Model file for the job. Use its own axes, mm. A direction names the side the tool comes from. Round coordinates to 2 decimals unless told otherwise and drop trailing zeros. Write each loop counter-clockwise with the first axis right and the second up, starting at its lowest first coordinate (ties: lowest second). Pieces come first, ordered by that corner, then holes.
Autodesk Inventor part; units mm, degrees
ref_plane "YZ Plane" through (0, 0, 0) normal (1, 0, 0) x (0, 1, 0)
ref_plane "XZ Plane" through (0, 0, 0) normal (0, 1, 0) x (-1, 0, 0)
ref_plane "XY Plane" through (0, 0, 0) normal (0, 0, 1) x (1, 0, 0)
sketch "Sketch1" plane through (0, 0, 0) normal (0, 0, 1) x (1, 0, 0)
  line L0 (0, 0) -> (50, 0)
  line L1 (50, 0) -> (50, 50)
  line L2 (50, 50) -> (0, 50)
  line L3 (0, 13.5853) -> (5.2, 11.6926)
  line L4 (5.2, 11.6926) -> (5.2, 22.0926)
  line L5 (5.2, 22.0926) -> (0, 20.2)
  line L6 (0, 50) -> (0, 20.2)
  line L7 (0, 13.5853) -> (0, 0)
  line L8 (0, 40.2) -> (5.2, 42.0926)
  line L9 (5.2, 42.0926) -> (5.2, 31.6926)
  line L10 (5.2, 31.6926) -> (0, 33.5853)
  dimension "d0" = 50
  dimension "d1" = 50
  dimension "d2" = 50
  dimension "d8" = 10.4
  dimension "d9" = 70
  dimension "d10" = 70
  dimension "d11" = 20.2
  dimension "d12" = 5.2
  dimension "d13" = 5.2
  dimension "d14" = 10.4
  dimension "d15" = 40.2
  dimension "d16" = 70
  dimension "d17" = 70
  dimension "d18" = 6.6147
  dimension "d19" = 6.6147
  dimension "d26" = 13.5853
extrude "Extrusion1" add sketch "Sketch1" along normal blind 10 contours L7 L3 L4 L5 L6 L10 L9 L8 L2 L1 L0
sketch "Sketch2" plane through (0, 0, 10) normal (0, 0, 1) x (1, 0, 0)
  line L0 (0, 13.5853) -> (0, 0)
  line L1 (0, 0) -> (50, 0)
  line L2 (50, 0) -> (50, 6.2593)
  line L3 (50, 0) -> (50, 50)
  line L4 (0, 0) -> (0, 6.2593)
  line L5 (0, 0) -> (50, 0)
  line L6 (0, 6.2593) -> (50, 6.2593)
  circle A0 centre (25, 25) radius 2.8
  dimension "d23" = 5.6
extrude "Extrusion2" add sketch "Sketch2" along normal blind 45
sketch "Sketch3" plane through (0, 0, 0) normal (0, 0, -1) x (-1, 0, 0)
  line L0 (0, 6.2593) -> (-50, 6.2593)
  line L1 (0, 6.2593) -> (-50, 6.2593)
  line L2 (0, 0) -> (-50, 0)
  line L3 (-50, 6.2593) -> (-50, 0)
  line L4 (-50, 0) -> (0, 0)
  line L5 (0, 6.2593) -> (0, 0)
  line L6 (0, 0) -> (0, 6.2593)
extrude "Extrusion3" add sketch "Sketch3" along normal blind 20
fillet "Fillet1" radius 5 1 edges at (25, 6.2593, 0)
fillet "Fillet2" radius 5 1 edges at (25, 50, 0)
fillet "Fillet3" radius 5 1 edges at (25, 50, 10)
fillet "Fillet4" radius 1 1 edges at (22.2, 25, 55)
properties part number "SpoolWinderBase"
1) Wall check: probe 1 along Y at (x, z) = (25, 41); probe 2 along X at (y, z) = (15, 3.5); probe 3 along Y at (x, z) = (45, 44.5). Give the ranges that are in metal, low to high.
2) Cut at B-B on y = 25. List the corners of the cut face in (x, z), and give its area (3 significant figures).
3) Which spindle directions (+Z, -Z, +X, -X, +Y, -Y) get a long thin tool onto all of the face, cutting with end or side? Do faces 1 (the face through (22.2, 24.9, 31.7)), 2 (the face through (2.64, 21.16, 4.93)), 3 (the face through (25, 3, -20)), 4 (the face through (25, 28, 0)). Say none if no direction does.
4) Pull direction Y, two halves, no side cores. Call faces 5 (the face through (25, 48, 9)), 6 (the face through (2.564, 12.652, 4.93)), 7 (the face through (25, 0, 18)), 8 (the face through (0, 27, 5)): released by +Y, released by -Y, zero draft, split by the parting line, or undercut.
5) Flat gauge pins, fed straight in: pin 1 Ø5 at (x, y) = (37, 37.5) entering from -Z; pin 2 Ø11 at (y, z) = (37.5, 4) entering from -X; pin 3 Ø5 at (x, z) = (15.5, 8.5) entering from +Y; pin 4 Ø3 at (x, y) = (35, 36) entering from +Z. Where does each tip first touch, or does it go through?
6) Cut at D-D on y = 37.5. List the corners of the cut face in (x, z), and give its area (3 significant figures).
Result sheet:
1. probe 1: y = 0 to 6.26, 22.2 to 27.8
1. probe 2: x = 5.2 to 50
1. probe 3: y = 0 to 6.26
2. outline: (0, 0) - (50, 0) - (50, 10) - (27.8, 10) - (27.8, 54) arc R1 ccw to (26.8, 55) - (23.2, 55) arc R1 ccw to (22.2, 54) - (22.2, 10) - (0, 10) - close
2. area: 752 mm2
3. face 1: +Z
3. face 2: +Z, -Z
3. face 3: -Z, +X, -X, +Y, -Y
3. face 4: -Z, +X, -X, +Y
4. face 5: released by +Y
4. face 6: undercut
4. face 7: released by -Y
4. face 8: zero draft
5. pin 1: stops at z = 0
5. pin 2: stops at x = 0
5. pin 3: stops at y = 49.9
5. pin 4: stops at z = 10
6. outline: (5.2, 0) - (50, 0) - (50, 10) - (5.2, 10) - close
6. area: 448 mm2
